from build123d import *

# Parameters (mm, degrees)
F0_W      = 200
F0_H      = 200
F1_DEPTH  = 15
F3_DEPTH  = 5
F2_W      = 200
F2_H      = 0.5
F4_DEPTH  = 4
F5_W      = 0.5
F5_H      = 200
F6_DEPTH  = 4
F8_DEPTH  = 4
F9_R      = 2.5
F10_DEPTH = 1.2
F11_R     = 2.5
F12_DEPTH = 2
F13_R     = 2.5
F14_DEPTH = 2
F15_SIZE  = 2
F16_R     = 2.5
F17_DEPTH = 2
F18_R     = 2.5
F19_DEPTH = 2


with BuildPart() as f1:
    # F0 (on Front) → F1 (new body)
    with BuildSketch(Plane.XZ):
        Rectangle(F0_W, F0_H)
    extrude(amount=F1_DEPTH)

    # F2 (on face) → F4 (cut)
    with BuildSketch(Plane.XZ.offset(15)):
        with Locations((0, 99.75)):
            Rectangle(F2_W, F2_H)
        with Locations((0, 59.75)):
            Rectangle(F2_W, F2_H)
        with Locations((0, 19.75)):
            Rectangle(F2_W, F2_H)
        with Locations((0, -20.25)):
            Rectangle(F2_W, F2_H)
        with Locations((0, -60.25)):
            Rectangle(F2_W, F2_H)
        with Locations((0, -100.25)):
            Rectangle(F2_W, F2_H)
    extrude(amount=-F4_DEPTH, mode=Mode.SUBTRACT)

    # F5 (on face) → F6 (cut)
    with BuildSketch(Plane.XZ.offset(15)):
        with Locations((-99.75, 0)):
            Rectangle(F5_W, F5_H)
        with Locations((-59.75, 0)):
            Rectangle(F5_W, F5_H)
        with Locations((-19.75, 0)):
            Rectangle(F5_W, F5_H)
        with Locations((20.25, 0)):
            Rectangle(F5_W, F5_H)
        with Locations((60.25, 0)):
            Rectangle(F5_W, F5_H)
        with Locations((100.25, 0)):
            Rectangle(F5_W, F5_H)
    extrude(amount=-F6_DEPTH, mode=Mode.SUBTRACT)

    # F7 (on face) → F8 (cut)
    with BuildSketch(Plane.XZ.offset(15)):
        Polygon((-100, -99.5), (-100, -100), (99.5, -100), (100, -100), (100, -99.5), (100, 99.5), (99.5, 99.5), (99.5, -99.5), align=None)
    extrude(amount=-F8_DEPTH, mode=Mode.SUBTRACT)

    # F9 (on face) → F10 (cut)
    with BuildSketch(Plane.XZ.offset(15)):
        with Locations((-79.75, 79.75)):
            Circle(F9_R)
        with Locations((-79.75, 40.25)):
            Circle(F9_R)
        with Locations((-79.75, 0.75)):
            Circle(F9_R)
        with Locations((-79.75, -38.75)):
            Circle(F9_R)
        with Locations((-79.75, -78.25)):
            Circle(F9_R)
        with Locations((-40.25, 79.75)):
            Circle(F9_R)
        with Locations((-40.25, 40.25)):
            Circle(F9_R)
        with Locations((-40.25, 0.75)):
            Circle(F9_R)
        with Locations((-40.25, -38.75)):
            Circle(F9_R)
        with Locations((-40.25, -78.25)):
            Circle(F9_R)
        with Locations((-0.75, 79.75)):
            Circle(F9_R)
        with Locations((-0.75, 40.25)):
            Circle(F9_R)
        with Locations((-0.75, 0.75)):
            Circle(F9_R)
        with Locations((-0.75, -38.75)):
            Circle(F9_R)
        with Locations((-0.75, -78.25)):
            Circle(F9_R)
        with Locations((38.75, 79.75)):
            Circle(F9_R)
        with Locations((38.75, 40.25)):
            Circle(F9_R)
        with Locations((38.75, 0.75)):
            Circle(F9_R)
        with Locations((38.75, -38.75)):
            Circle(F9_R)
        with Locations((38.75, -78.25)):
            Circle(F9_R)
        with Locations((78.25, 79.75)):
            Circle(F9_R)
        with Locations((78.25, 40.25)):
            Circle(F9_R)
        with Locations((78.25, 0.75)):
            Circle(F9_R)
        with Locations((78.25, -38.75)):
            Circle(F9_R)
        with Locations((78.25, -78.25)):
            Circle(F9_R)
    extrude(amount=-F10_DEPTH, mode=Mode.SUBTRACT)



with BuildPart() as f3:
    # F0 (on Front) → F3 (new body)
    with BuildSketch(Plane.XZ):
        Rectangle(F0_W, F0_H)
    extrude(amount=F3_DEPTH)


with BuildPart() as f1_1:
    add(f1.part)

    add(f3.part)  # F12 merges F3
    # F11 (on face) → F12 (join)
    with BuildSketch(Plane.YZ.offset(100)):
        with Locations((-5.5, -74.5)):
            Circle(F11_R)
        with Locations((-5.5, 74.5)):
            Circle(F11_R)
    extrude(amount=F12_DEPTH)

    # F13 (on face) → F14 (join)
    with BuildSketch(Plane(origin=(0, 0, -100), x_dir=(1, 0, 0), z_dir=(0, 0, -1))):
        with Locations((-74.5, 5.5)):
            Circle(F13_R)
        with Locations((74.5, 5.5)):
            Circle(F13_R)
    extrude(amount=F14_DEPTH)

    # F15
    f15_edges = [f1_1.edges().sort_by_distance(p)[0] for p in [
        (0, 0, -100),
        (100, 0, 0),
        (0, 0, 100),
        (-100, 0, 0),
    ]]
    chamfer(f15_edges, length=F15_SIZE)

    # F16 (on face) → F17 (join)
    with BuildSketch(Plane(origin=(-100, 0, 0), x_dir=(0, -1, 0), z_dir=(-1, 0, 0))):
        with Locations((5.5, -74.5)):
            Circle(F16_R)
        with Locations((5.5, 74.5)):
            Circle(F16_R)
    extrude(amount=F17_DEPTH)

    # F18 (on face) → F19 (join)
    with BuildSketch(Plane.XY.offset(100)):
        with Locations((74.5, -5.5)):
            Circle(F18_R)
        with Locations((-74.5, -5.5)):
            Circle(F18_R)
    extrude(amount=F19_DEPTH)


solid = f1_1.part
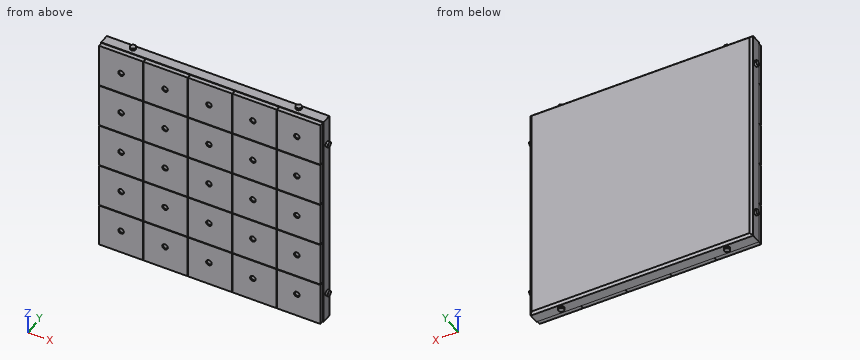
Model file for the job. Use its own axes, mm. Give positions to 0.01 mm unless a question says otherwise; leave off trailing zeros. Order: outer loops, then holes, each group sorted by start corner. A loop starts at its lowest first (then second) coordinate and runs counter-clockwise, first axis right, second up. Notation, with made-up numbers: (15.25, -10.75) - (24.25, -10.75) arc R20 cw to (24.25, 20.25) - close; hole circle Ø9 at (58, -30). An arc over 180 degrees is marked (long way). Write item = value, one per line. Start each with the question number.
1. Drop flat-ended pins along their axis: P1, Ø1.2, axis at y = -12.5, z = 42.5, coming from the +X side; P2, Ø4.5, axis at x = -45.5, y = -13.5, coming from the +Z side; P3, Ø1.5, axis at x = -0.5, z = 0, coming from the -Y side. Give the stop position or say it passes through.
2. Cut at A-A, the plane z = -33. List the corners of the cut face in (x, y), and give its area (3 significant figures).
3. Probe line 1 along Z through (x, y) = (26.5, -13.25); line 2 along X through (y, z) = (-13.75, 48); line 3 along Z through (x, y) = (-49.5, -9). List the from-to ranges inside material, lowest first.
4. Cut at B-B, the plane x = -8. List the corners of the cut face in (y, z), and give its area (3 significant figures).
Taken from the geometry:
q1.P1 = 99.5
q1.P2 = 99.5
q1.P3 = -13.8
q2.outline = (-100, -11) - (-99.5, -11) - (-99.5, -15) - (-60, -15) - (-60, -11) - (-59.5, -11) - (-59.5, -15) - (-20, -15) - (-20, -11) - (-19.5, -11) - (-19.5, -15) - (20, -15) - (20, -11) - (20.5, -11) - (20.5, -15) - (60, -15) - (60, -11) - (60.5, -11) - (60.5, -15) - (99.5, -15) - (99.5, -11) - (100, -11) - (100, -2) - (98, 0) - (-98, 0) - (-100, -2) - close
q2.area = 2,980 mm²
q3.line_1 = -99.5 to -60.5, -60 to -20.5, -20 to 19.5, 20 to 59.5, 60 to 99.5
q3.line_2 = -99.5 to -60, -59.5 to -20, -19.5 to 20, 20.5 to 60, 60.5 to 99.5
q3.line_3 = -100 to 100
q4.outline = (-15, -99.5) - (-11, -99.5) - (-11, -100) - (-2, -100) - (0, -98) - (0, 98) - (-2, 100) - (-11, 100) - (-11, 99.5) - (-15, 99.5) - (-15, 60) - (-11, 60) - (-11, 59.5) - (-15, 59.5) - (-15, 20) - (-11, 20) - (-11, 19.5) - (-15, 19.5) - (-15, -20) - (-11, -20) - (-11, -20.5) - (-15, -20.5) - (-15, -60) - (-11, -60) - (-11, -60.5) - (-15, -60.5) - close
q4.area = 2,980 mm²
